Check sheet for the modelled part. Datum: model origin and axes. Units: mm. A direction names the side the tool comes from. Coordinates: 2 decimals unless noted, no trailing zeros. Order: outer loops, then holes, each group sorted by start corner. A loop starts at its lowest first (then second) coordinate and runs counter-clockwise, first axis right, second up.
from build123d import *

# Parameters (mm, degrees)
ESQUISSE1_W             = 51
ESQUISSE1_H             = 50
BOSS_EXTRU_1_DEPTH      = 2.5
ESQUISSE2_W             = 10
ESQUISSE2_H             = 2.9
BOSS_EXTRU_2_DEPTH      = 15
ESQUISSE3_W             = 51
ESQUISSE3_H             = 2.9
ESQUISSE3_H_2           = 3
BOSS_EXTRU_3_DEPTH      = 3
ESQUISSE4_R             = 1.5
ENL_V_MAT_EXTRU_1_DEPTH = 46.937457483


with BuildPart() as part:
    # Esquisse1 → Boss.-Extru.1 (new body)
    with BuildSketch(Plane.XY):
        Rectangle(ESQUISSE1_W, ESQUISSE1_H)
    extrude(amount=BOSS_EXTRU_1_DEPTH)

    # Esquisse2 → Boss.-Extru.2 (add)
    with BuildSketch(Plane(origin=(0, 0, 0), x_dir=(-1, 0, 0), z_dir=(0, 0, -1))):
        with Locations((-30.5, 23.55)):
            Rectangle(ESQUISSE2_W, ESQUISSE2_H)
        with Locations((30.5, 23.55)):
            Rectangle(ESQUISSE2_W, ESQUISSE2_H)
    extrude(amount=-BOSS_EXTRU_2_DEPTH)

    # Esquisse3 → Boss.-Extru.3 (add)
    with BuildSketch(Plane.XY.offset(2.5)):
        with Locations((0, 23.55)):
            Rectangle(ESQUISSE3_W, ESQUISSE3_H)
        with Locations((0, -23.5)):
            Rectangle(ESQUISSE3_W, ESQUISSE3_H_2)
    extrude(amount=BOSS_EXTRU_3_DEPTH)

    # Esquisse4 → Enlèv. mat.-Extru.1 (cut, through all)
    with BuildSketch(Plane(origin=(0, 0, 0), x_dir=(-1, 0, 0), z_dir=(0, 0, -1))):
        with Locations((18.506042036, -12.531837257)):
            Circle(ESQUISSE4_R)
        with Locations((-18.493956712, -12.531832115)):
            Circle(ESQUISSE4_R)
        with Locations((-18.505955671, 15.468170274)):
            Circle(ESQUISSE4_R)
        with Locations((18.506042036, 15.468170274)):
            Circle(ESQUISSE4_R)
    extrude(amount=-ENL_V_MAT_EXTRU_1_DEPTH, mode=Mode.SUBTRACT)


solid = part.part
(1) Thickness scan on probe 1 along Z at (x, y) = (-18.5, -19); probe 2 along Y at (x, z) = (26, 13.75). Record the ranges inside material, lowest first.
Filled in:
probe 1: z = 0 to 2.5
probe 2: y = 22.1 to 25
(2) Cross-section at C-C (y = 10). Enter the section's corners in (x, z).
Filled in:
outline: (-25.5, 0) - (25.5, 0) - (25.5, 2.5) - (-25.5, 2.5) - close
(3) Release check for a two-part mould opening along X. For faces 4 (the flat face through (35.5, 24, 7)), 5 (the cylindrical face through (19.993, -12.466, 1.232)), 6 (the flat face through (0, 0, 2.5)) record: +X half, -X half, draft (parallel to the pull), parting line (faces both ways), or undercut.
Filled in:
face 4: +X half
face 5: undercut
face 6: draft
(4) Tool access check on faces 1 (the flat face through (0, 24, 5.5)), 2 (the flat face through (25.5, -2, 1)), 3 (the flat face through (0, -22, 4)). Record the directions out of +Z, -Z, +X, -X, +Y, -Y that give a thin tool (end or side, any length) a straight path to the whole face; none if there is none.
Filled in:
face 1: +Z, +Y, -Y
face 2: +Z, -Z, +X, -Y
face 3: +Z, +X, -X
(5) Go/stop test with flat-tipped pins: P1, Ø1.5, axis at y = 0.5, z = 2.5, coming from the -X side; P2, Ø3, axis at x = 0.5, y = 23.5, coming from the +Z side; P3, Ø6, axis at y = -12, z = 5, coming from the +X side. Record where each tip stops, or that it passes through.
Filled in:
P1: stops at x = -25.5
P2: stops at z = 5.5
P3: stops at x = 25.5
(6) Cross-section at A-A (z = 6.75). Enter the section's corners in (x, y).
Filled in:
outline: (-35.5, 22.1) - (-25.5, 22.1) - (-25.5, 25) - (-35.5, 25) - close; (25.5, 22.1) - (35.5, 22.1) - (35.5, 25) - (25.5, 25) - close
(7) Cross-section at B-B (x = 18.5). Enter the section's corners in (y, z).
Filled in:
outline: (-25, 0) - (-14.03, 0) - (-14.03, 2.5) - (-22, 2.5) - (-22, 5.5) - (-25, 5.5) - close; (-11.03, 0) - (13.97, 0) - (13.97, 2.5) - (-11.03, 2.5) - close; (16.97, 0) - (25, 0) - (25, 5.5) - (22.1, 5.5) - (22.1, 2.5) - (16.97, 2.5) - close
(8) Cross-section at D-D (x = 31). Enter the section's corners in (y, z), and give its area (3 significant figures).
Filled in:
outline: (22.1, 0) - (25, 0) - (25, 15) - (22.1, 15) - close
area: 43.5 mm2
